from build123d import *

# Parameters (mm, degrees)
SKETCH1_W           = 50.8
SKETCH1_H           = 25.4
BOSS_EXTRUDE1_DEPTH = 609.6
SKETCH2_W           = 44.45
SKETCH2_H           = 19.05
CUT_EXTRUDE1_DEPTH  = 635
SKETCH6_R           = 14.2875
CUT_EXTRUDE5_DEPTH  = 3.175
SKETCH7_R           = 14.2875
CUT_EXTRUDE6_DEPTH  = 3.175
SKETCH8_R           = 4.7625
CUT_EXTRUDE7_DEPTH  = 25.4


with BuildPart() as part:
    # Sketch1 → Boss-Extrude1 (new body)
    with BuildSketch(Plane.XY):
        with Locations((25.4, 12.7)):
            Rectangle(SKETCH1_W, SKETCH1_H)
    extrude(amount=BOSS_EXTRUDE1_DEPTH)

    # Sketch2 → Cut-Extrude1 (cut)
    with BuildSketch(Plane(origin=(0, 0, 0), x_dir=(-1, 0, 0), z_dir=(0, 0, -1))):
        with Locations((-25.4, 12.7)):
            Rectangle(SKETCH2_W, SKETCH2_H)
    extrude(amount=-CUT_EXTRUDE1_DEPTH, mode=Mode.SUBTRACT)

    # Sketch6 → Cut-Extrude5 (cut)
    with BuildSketch(Plane(origin=(0, 25.4, 0), x_dir=(1, 0, 0), z_dir=(0, 1, 0))):
        with Locations((25.4, -25.4)):
            Circle(SKETCH6_R)
    extrude(amount=-CUT_EXTRUDE5_DEPTH, mode=Mode.SUBTRACT)

    # Sketch7 → Cut-Extrude6 (cut)
    with BuildSketch(Plane(origin=(0, 25.4, 0), x_dir=(1, 0, 0), z_dir=(0, 1, 0))):
        with Locations((25.4, -584.2)):
            Circle(SKETCH7_R)
    extrude(amount=-CUT_EXTRUDE6_DEPTH, mode=Mode.SUBTRACT)

    # Sketch8 → Cut-Extrude7 (cut)
    with BuildSketch(Plane(origin=(0, 0, 0), x_dir=(-1, 0, 0), z_dir=(0, -1, 0))):
        with Locations((-25.4, -558.8)):
            Circle(SKETCH8_R)
    extrude(amount=-CUT_EXTRUDE7_DEPTH, mode=Mode.SUBTRACT)


solid = part.part
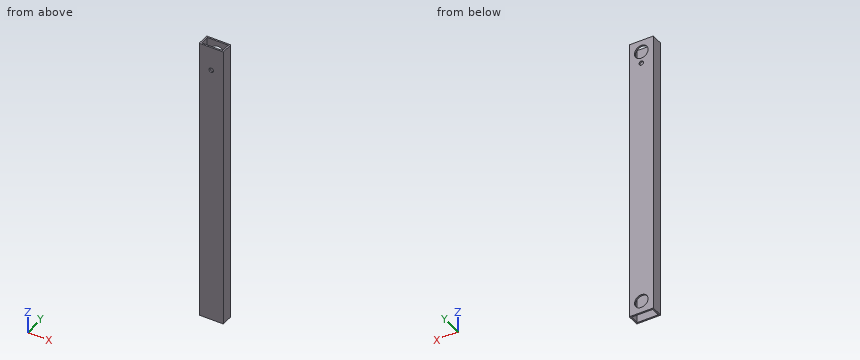
Geometry: final body of the model. Coordinates: model frame, mm. Give positions to 0.01 mm unless a question says otherwise; leave off trailing zeros. Loops run counter-clockwise (first coordinate to the right, second up) from the corner with the lowest first, then second, coordinate; pieces in that order, holes last. Notation, with made-up numbers: (3, 82) -> (15, 82) arc R22 cw to (15, 118) -> close; hole circle Ø8 at (78.25, -9.75). An arc over 180 degrees is marked (long way). Put each result on its own line as item: value.
1. Cut plane B-B (y = 10.5). Return the cut outline in (x, z) (3 decimals).
Taken from the geometry:
outline: (0, 0) -> (3.175, 0) -> (3.175, 609.6) -> (0, 609.6) -> close; (47.625, 0) -> (50.8, 0) -> (50.8, 609.6) -> (47.625, 609.6) -> close
2. Cut plane C-C (z = 25.4). Return the cut outline in (x, y) (1 decimal).
Taken from the geometry:
outline: (0, 0) -> (50.8, 0) -> (50.8, 25.4) -> (39.7, 25.4) -> (39.7, 22.2) -> (47.6, 22.2) -> (47.6, 3.2) -> (3.2, 3.2) -> (3.2, 22.2) -> (11.1, 22.2) -> (11.1, 25.4) -> (0, 25.4) -> close
3. Cut plane A-A (z = 454). Return the cut outline in (x, y) (3 decimals), plus the area to 3 significant figures.
Taken from the geometry:
outline: (0, 0) -> (50.8, 0) -> (50.8, 25.4) -> (0, 25.4) -> close; hole (3.175, 3.175) -> (47.625, 3.175) -> (47.625, 22.225) -> (3.175, 22.225) -> close
area: 444 mm2
4. Pin query (flat end, axial travel): P1, Ø23, axis at x = 25.4, z = 584.2, coming from the +Y side (3 decimals). Return the tip coordinate at first contact, or that it passes through.
Taken from the geometry:
P1: stops at y = 3.175
5. Ray query, line 1 along Z through (x, y) = (25.4, 24.55); line 2 along X through (y, z) = (9.25, 501) (3 decimals); line 3 along X through (y, z) = (23.1, 558.8). Return the intervals inside material, ascending. Write a range as [from, to].
Taken from the geometry:
line 1: z = [0, 11.11], [39.69, 554.04], [563.56, 569.91], [598.49, 609.6]
line 2: x = [0, 3.175], [47.625, 50.8]
line 3: x = [0, 20.64], [30.16, 50.8]
